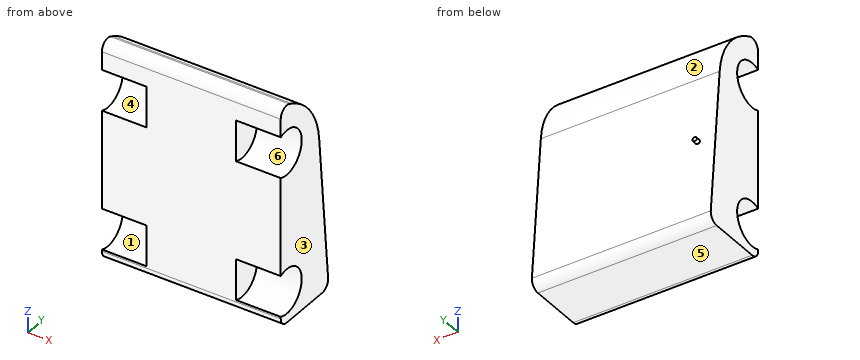
from build123d import *

# Parameters (mm, degrees)
BOSS_EXTRUDE1_DEPTH = 100
SKETCH3_R           = 25
CUT_EXTRUDE1_DEPTH  = 50
SKETCH4_R           = 2.5
BOSS_EXTRUDE2_DEPTH = 5


with BuildPart() as part:
    # Sketch2 → Boss-Extrude1 (new, symmetric)
    with BuildSketch(Plane(origin=(0, 0, 0), x_dir=(0, 0, -1), z_dir=(1, 0, 0))):
        with BuildLine():
            Line((-112.643906845, 14.257821235), (-110.645286598, 18.505070953))
            ThreePointArc((-110.645286598, 18.505070953), (-84.118524888, 49.993435328), (-45.444881226, 64.119137564))
            Line((-45.444881226, 64.119137564), (119.748610721, 79.017143226))
            ThreePointArc((119.748610721, 79.017143226), (127.392850703, 76.439367824), (130.646817248, 69.057563665))
            Line((130.646817248, 69.057563665), (130.646817248, 10))
            ThreePointArc((130.646817248, 10), (127.71788506, 2.928932188), (120.646817248, 0))
            Line((120.646817248, 0), (-103.595649647, 0))
            ThreePointArc((-103.595649647, 0), (-112.038937287, 4.641745263), (-112.643906845, 14.257821235))
        make_face()
    extrude(amount=BOSS_EXTRUDE1_DEPTH, both=True)

    # Sketch3 → Cut-Extrude1 (cut)
    with BuildSketch(Plane(origin=(100, 0, 0), x_dir=(0, 0, -1), z_dir=(1, 0, 0))):
        with Locations((-60.35749377, 10)):
            Circle(SKETCH3_R)
        with Locations((95.561704497, 10)):
            Circle(SKETCH3_R)
    cut_extrude1 = extrude(amount=-CUT_EXTRUDE1_DEPTH, mode=Mode.SUBTRACT)

    # Mirror1: Cut-Extrude1 across plane
    add(cut_extrude1.mirror(Plane(origin=(0, 0, 0), x_dir=(0, 0, 1), z_dir=(1, 0, 0))), mode=Mode.SUBTRACT)

    # Sketch4 → Boss-Extrude2 (add)
    with BuildSketch(Plane(origin=(0, 67.667230134, 6.102581681), x_dir=(1, 0, 0), z_dir=(0, 0.9959579561140941, 0.0898206527088083))):
        with Locations(Location((-80, 36.574402855, 0), (0, 0, 90))):
            Circle(SKETCH4_R)
    extrude(amount=BOSS_EXTRUDE2_DEPTH)


solid = part.part
Here's how the part is built. I have some questions about the finished solid (model axes, mm). Face numbers are marked on the shaded views. A direction names the side the tool comes from. Round coordinates to 2 decimals unless told otherwise and drop trailing zeros. Write each loop counter-clockwise with the first axis right and the second up, starting at its lowest first coordinate (ties: lowest second). Pieces come first, ordered by that corner, then holes. Notation, with made-up numbers: (83, 5.25) -> (104, 5.25) arc R19 cw to (104, 39.25) -> close; hole circle Ø10 at (46, 24). An arc over 180 degrees is marked (long way). One line per item, written item: value.
1) Suppose I cut it at A-A on x = 37.5. List the corners of the cut face in (y, z) for me, plus the area to 3 significant figures.
Filled sheet:
outline: (0, -120.65) arc R10 ccw to (10, -130.65) -> (69.06, -130.65) arc R10 ccw to (79.02, -119.75) -> (64.12, 45.44) arc R80 ccw to (18.51, 110.65) -> (14.26, 112.64) arc R10 ccw to (0, 103.6) -> close
area: 15,900 mm2
2) We'd pull the mould along Z, two halves only. Please class the marked faces 1, 2 and 3: released by +Z, released by -Z, zero draft, split by the parting line, or undercut.
Filled sheet:
face 1: undercut
face 2: released by +Z
face 3: zero draft
3) For the marked faces 4, 5 and 6, which set-ups out of +Z, -Z, +X, -X, +Y, -Y let a thin tool reach every point of the face, with its end or its side?
Filled sheet:
face 4: -X
face 5: -Z, +X, -X, +Y, -Y
face 6: +X
4) If I drill on line 1 (Z direction, x = 63.5, y = 10); line 2 (Z direction, x = -53.5, y = 14); line 3 (X direction, y = 3.5, z = -88.5), over which ranges is the centre line in solid material (lowest first)? Write a range as [from, to].
Filled sheet:
line 1: z = [-130.65, -120.56], [-70.56, 35.36], [85.36, 113.6]
line 2: z = [-130.65, -120.24], [-70.88, 35.68], [85.04, 112.76]
line 3: x = [-50, 50]
5) Suppose I cut it at B-B on z = 55.5. List the corners of the cut face in (x, y) for me, plus the area to 3 significant figures.
Filled sheet:
outline: (-100, 34.52) -> (-50, 34.52) -> (-50, 0) -> (50, 0) -> (50, 34.52) -> (100, 34.52) -> (100, 62.56) -> (-100, 62.56) -> close
area: 9,060 mm2
6) Suppose I cut it at D-D on z = 7. List the corners of the cut face in (x, y) for me.
Filled sheet:
outline: (-100, 0) -> (100, 0) -> (100, 67.59) -> (-100, 67.59) -> close
7) Suppose I cut it at C-C on y = 42.5. List the corners of the cut face in (x, z) for me.
Filled sheet:
outline: (-100, -130.65) -> (100, -130.65) -> (100, 93.3) -> (-100, 93.3) -> close
8) I'm going to push flat-ended pins straight in: pin 1 Ø1.5 at (x, y) = (33.5, 35.5) entering from +Z; pin 2 Ø4 at (x, z) = (-74.5, -96) entering from +Y; pin 3 Ø12 at (x, z) = (75.5, 84) entering from +Y. Where does each tip first touch, or does it pass through?
Filled sheet:
pin 1: stops at z = 100.46
pin 2: stops at y = 77.06
pin 3: stops at y = 53.87
